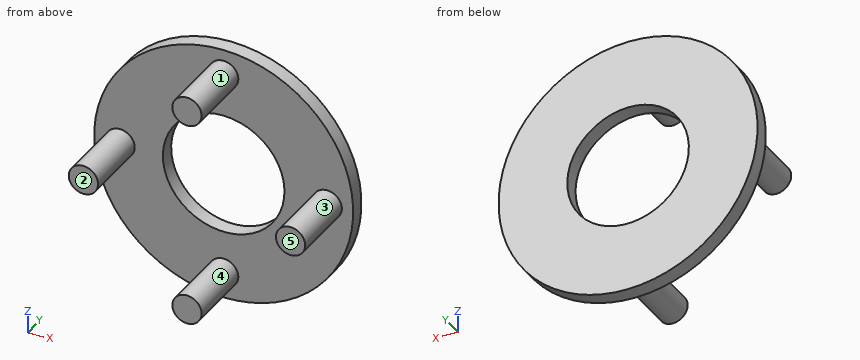
from build123d import *

# Parameters (mm, degrees)
SKETCH_1_R      = 57.5
SKETCH_1_R_2    = 27
EXTRUDE_2_DEPTH = 6.75
SKETCH_3_R      = 6.5
EXTRUDE_3_DEPTH = 30


with BuildPart() as part:
    # 草圖1 → 填料-伸長2 (new body)
    with BuildSketch(Plane(origin=(0, 0, 0), x_dir=(1, 0, 0), z_dir=(0, 1, 0))):
        with Locations(Location((0, 0, 0), (0, 0, 270))):
            Circle(SKETCH_1_R)
        with Locations(Location((0, 0, 0), (0, 0, 270))):
            Circle(SKETCH_1_R_2, mode=Mode.SUBTRACT)
    extrude(amount=EXTRUDE_2_DEPTH)

    # 草圖3 → 填料-伸長3 (add)
    with BuildSketch(Plane.XZ):
        with Locations(Location((0, 46, 0), (0, 0, 90))):
            Circle(SKETCH_3_R)
        with Locations(Location((0, -46, 0), (0, 0, 90))):
            Circle(SKETCH_3_R)
        with Locations(Location((-46, 0, 0), (0, 0, 90))):
            Circle(SKETCH_3_R)
        with Locations(Location((46, 0, 0), (0, 0, 90))):
            Circle(SKETCH_3_R)
    extrude(amount=EXTRUDE_3_DEPTH)


solid = part.part
Model file for the job. Use its own axes, mm. Face numbers are marked on the shaded views. A direction names the side the tool comes from. Coordinates: 2 decimals unless noted, no trailing zeros. Write each loop counter-clockwise with the first axis right and the second up, starting at its lowest first coordinate (ties: lowest second). Pieces come first, ordered by that corner, then holes. Notation, with made-up numbers: (42, 47.25) -> (64, 47.25) arc R30 cw to (64, 83.25) -> close; hole circle Ø11 at (68.25, 42). An arc over 180 degrees is marked (long way). One line per item, written item: value. Start each with the question number.
1) Slice it at C-C on x = 46. Write the cut outline in (y, z), then the cut area to 3 significant figures.
2) Slice it at A-A on z = 0. Write the cut outline in (x, y).
3) Slice it at B-B on x = 0. Write the cut outline in (y, z), then the cut area to 3 significant figures.
4) Flat gauge pins, fed straight in: pin 1 Ø12 at (x, z) = (-31, 8) entering from -Y; pin 2 Ø5 at (x, y) = (8, -10) entering from +Z; pin 3 Ø5 at (x, z) = (-8.5, -20.5) entering from +Y; pin 4 Ø6 at (x, y) = (-40, 0.5) entering from +Z. Where does each tip first touch, or does it go through?
5) Which spindle directions (+Z, -Z, +X, -X, +Y, -Y) get a long thin tool onto all of the face, cutting with end or side? Do the marked faces 4 and 5. Say none if no direction does.
6) Probe probe 1 along X at (y, z) = (2, 0); probe 2 along Y at (x, z) = (-28, -20); probe 3 along Z at (x, y) = (-6, -15.5). List the from-to ranges inside material, lowest first.
7) Pull direction X, two halves, no side cores. Call the marked faces 1, 2 and 3: +X half, -X half, draft (parallel to the pull), parting line (faces both ways), or undercut.
8) Slice it at D-D on y = -7.5. Write the cut outline in (x, z).
Answers follow:
1. outline: (-30, -6.5) -> (0, -6.5) -> (0, -34.5) -> (6.75, -34.5) -> (6.75, 34.5) -> (0, 34.5) -> (0, 6.5) -> (-30, 6.5) -> close
1. area: 856 mm2
2. outline: (-57.5, 0) -> (-52.5, 0) -> (-52.5, -30) -> (-39.5, -30) -> (-39.5, 0) -> (-27, 0) -> (-27, 6.75) -> (-57.5, 6.75) -> close; (27, 0) -> (39.5, 0) -> (39.5, -30) -> (52.5, -30) -> (52.5, 0) -> (57.5, 0) -> (57.5, 6.75) -> (27, 6.75) -> close
3. outline: (-30, -52.5) -> (0, -52.5) -> (0, -57.5) -> (6.75, -57.5) -> (6.75, -27) -> (0, -27) -> (0, -39.5) -> (-30, -39.5) -> close; (-30, 39.5) -> (0, 39.5) -> (0, 27) -> (6.75, 27) -> (6.75, 57.5) -> (0, 57.5) -> (0, 52.5) -> (-30, 52.5) -> close
3. area: 1,190 mm2
4. pin 1: y = 0
4. pin 2: z = 49.46
4. pin 3: through
4. pin 4: z = 44.01
5. face 4: -Y
5. face 5: +Z, -Z, +X, -X, -Y
6. probe 1: -57.5 to -27, 27 to 57.5
6. probe 2: 0 to 6.75
6. probe 3: -48.5 to -43.5, 43.5 to 48.5
7. face 1: parting line
7. face 2: draft
7. face 3: undercut
8. outline: circle Ø13 at (-46, 0); circle Ø13 at (0, -46); circle Ø13 at (0, 46); circle Ø13 at (46, 0)
